The model under review builds one solid part; all positions refer to its coordinate system, in mm. Round coordinates to 2 decimals unless told otherwise and drop trailing zeros. Order: outer loops, then holes, each group sorted by start corner. A loop starts at its lowest first (then second) coordinate and runs counter-clockwise, first axis right, second up. Notation, with made-up numbers: M 14,58.25 L 64,58.25 A6 cw 64,69.25 Z; hole C 70.5,-18.5 d1. An arc over 180 degrees is marked long. Answer as a JSON object with one key per item and string values. Group by question number.
1. Add section D-D on z = 11.5. State the section outline as (x, y) points, and give its area (3 significant figures).
2. Add section C-C on x = 50. State the section outline as (y, z) points, and give its area (3 significant figures).
3. Add section A-A on x = 13.5. State the section outline as (y, z) points, and give its area (3 significant figures).
4. Clearance check with a flat-ended pin moving along its axis: P1, Ø0.9, axis at x = 56.5, y = -1.5, coming from the +Z side. State where the tip first meets the part, or that it passes through.
5. Add section B-B on z = 21.5. State the section outline as (x, y) points.
6. To check wall thickness, follow probe 1 along Z at (x, y) = (59.5, -1.9); probe 2 along X at (y, z) = (-2.4, 17); probe 3 along Z at (x, y) = (19, -0.1). State the ranges of each line that lie inside material, in increasing order. Write a range as [from, to].
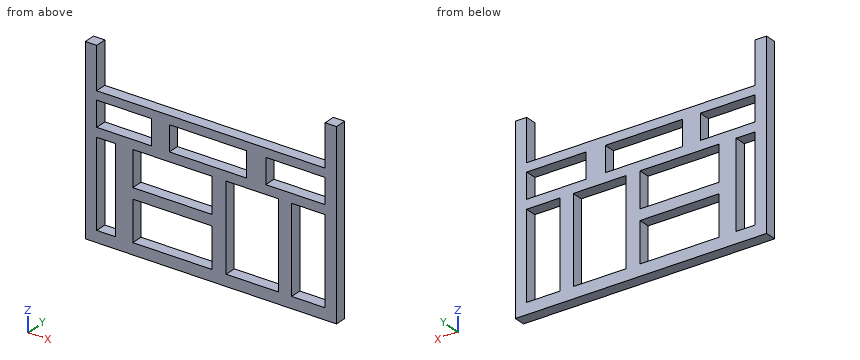
```python
from build123d import *

# Parameters (mm, degrees)
F1_DEPTH = 60
F2_W     = 5.0666704774
F2_H     = 6.6256467253
F2_H_2   = 1.0133311152
F2_W_2   = 4.6769259498
F2_H_3   = 1.2471787632
F2_H_4   = 1.4030765742
F2_W_3   = 3.4297443926
F2_H_5   = 23.8523234148
F2_H_6   = 0.8574351668
F2_W_4   = 4.5210286044
F2_H_7   = 1.0133348405
F2_W_5   = 3.7415400147
F2_W_6   = 20.7343716174
F2_H_8   = 2.8061550111
F2_W_7   = 1.1692317203
F2_W_8   = 1.4030784369
F3_DEPTH = 3
F4_W     = 106.1131954193
F4_H     = 74.4311399758
F5_DEPTH = 57


with BuildPart() as f1:
    # F0 (on Front) → F1 (new body)
    with BuildSketch(Plane.XZ):
        Polygon((60, 0), (0, 0), (0, 45), (-3, 45), (-3, -3), (63, -3), (63, 45), (60, 45), align=None)
    extrude(amount=F1_DEPTH)

    # F2 (on Front) → F3 (join)
    with BuildSketch(Plane.XZ):
        Polygon((60.8672574162, 31.6860154271), (60.8672574162, 33.9465290308), (-0.9461171576, 33.9465290308), (-0.9461171576, 31.6860154271), (14.4097907469, 31.6860154271), (14.4097907469, 32.9331941903), (19.0867166966, 32.9331941903), (19.0867166966, 31.6860154271), (39.3533967435, 31.6860154271), (39.3533967435, 32.6993465424), (44.4200672209, 32.6993465424), (44.4200672209, 31.6860154271), align=None)
        with Locations((41.8867319822, 28.3731920645)):
            Rectangle(F2_W, F2_H)
        with Locations((41.8867319822, 32.1926809847)):
            Rectangle(F2_W, F2_H_2)
        with Locations((16.7482537217, 32.3096048087)):
            Rectangle(F2_W_2, F2_H_3)
        with Locations((16.7482537217, 28.3731920645)):
            Rectangle(F2_W_2, F2_H)
        with Locations((41.8867319822, 24.3588304147)):
            Rectangle(F2_W, F2_H_4)
        Polygon((62.0364882052, 25.0603687018), (44.4200672209, 25.0603687018), (44.4200672209, 23.6572921276), (39.3533967435, 23.6572921276), (39.3533967435, 25.0603687018), (19.0867166966, 25.0603687018), (19.0867166966, 23.6572921276), (14.4097907469, 23.6572921276), (14.4097907469, 25.0603687018), (-2.1932963282, 25.0603687018), (-2.1932963282, 22.6439572871), (4.9779904075, 22.6439572871), (4.9779904075, 23.6572921276), (9.4990190119, 23.6572921276), (9.4990190119, 22.6439572871), (30.2333906293, 22.6439572871), (30.2333906293, 23.5013924539), (33.974930644, 23.5013924539), (33.974930644, 22.6439572871), (47.7718636394, 22.6439572871), (47.7718636394, 23.5013924539), (51.201608032, 23.5013924539), (51.201608032, 22.6439572871), (62.0364882052, 22.6439572871), align=None)
        with Locations((16.7482537217, 24.3588304147)):
            Rectangle(F2_W_2, F2_H_4)
        with Locations((49.4867358357, 10.7177955797)):
            Rectangle(F2_W_3, F2_H_5)
        with Locations((49.4867358357, 23.0726748705)):
            Rectangle(F2_W_3, F2_H_6)
        with Locations((7.2385047097, 23.1506247073)):
            Rectangle(F2_W_4, F2_H_7)
        Polygon((9.4990190119, 22.6439572871), (4.9779904075, 22.6439572871), (4.9779904075, -1.2083661277), (9.4990190119, -1.2083661277), (9.4990190119, 10.5618983507), (8.3297872916, 10.5618983507), (8.3297872916, 13.3680533618), (9.4990190119, 13.3680533618), align=None)
        Polygon((33.974930644, -1.2083661277), (33.974930644, 22.6439572871), (30.2333906293, 22.6439572871), (30.2333906293, 13.3680533618), (31.6364690661, 13.3680533618), (31.6364690661, 10.5618983507), (30.2333906293, 10.5618983507), (30.2333906293, -1.2083661277), align=None)
        with Locations((32.1041606367, 23.0726748705)):
            Rectangle(F2_W_5, F2_H_6)
        with Locations((19.8662048206, 11.9649758562)):
            Rectangle(F2_W_6, F2_H_8)
        with Locations((8.9144031517, 11.9649758562)):
            Rectangle(F2_W_7, F2_H_8)
        with Locations((30.9349298477, 11.9649758562)):
            Rectangle(F2_W_8, F2_H_8)
    extrude(amount=F3_DEPTH)

    # F4 (on face) → F5 (cut, through all)
    with BuildSketch(Plane.XZ.offset(60)):
        with Locations((33.7975099683, 20.7829978317)):
            Rectangle(F4_W, F4_H)
    extrude(amount=-F5_DEPTH, mode=Mode.SUBTRACT)


solid = f1.part
```
Recorded:
{
 "1": {"outline": "M -3,-3 L 0,-3 L 0,0 L -3,0 Z; M 4.98,-3 L 33.97,-3 L 33.97,0 L 4.98,0 Z; M 47.77,-3 L 51.2,-3 L 51.2,0 L 47.77,0 Z; M 60,-3 L 63,-3 L 63,0 L 60,0 Z", "area": "115 mm²"},
 "2": {"outline": "M -3,-3 L 0,-3 L 0,25.06 L -3,25.06 Z; M -3,31.69 L 0,31.69 L 0,33.95 L -3,33.95 Z", "area": "91.0 mm²"},
 "3": {"outline": "M -3,-3 L 0,-3 L 0,0 L -3,0 Z; M -3,10.56 L 0,10.56 L 0,13.37 L -3,13.37 Z; M -3,22.64 L 0,22.64 L 0,25.06 L -3,25.06 Z; M -3,31.69 L 0,31.69 L 0,33.95 L -3,33.95 Z", "area": "31.4 mm²"},
 "4": {"P1": "stops at z = 33.95"},
 "5": {"outline": "M -3,-3 L 0,-3 L 0,0 L -3,0 Z; M 4.98,-3 L 9.5,-3 L 9.5,0 L 4.98,0 Z; M 30.23,-3 L 33.97,-3 L 33.97,0 L 30.23,0 Z; M 47.77,-3 L 51.2,-3 L 51.2,0 L 47.77,0 Z; M 60,-3 L 63,-3 L 63,0 L 60,0 Z"},
 "6": {"probe 1": "z = [-3, 0], [22.64, 25.06], [31.69, 33.95]", "probe 2": "x = [-3, 0], [4.98, 9.5], [30.23, 33.97], [47.77, 51.2], [60, 63]", "probe 3": "z = [-3, 0], [10.56, 13.37], [22.64, 33.95]"}
}
